```python
from build123d import *

# Parameters (mm, degrees)
F1_DEPTH = 44.45
F2_T     = -2.54
F4_DEPTH = 3.81
F5_R     = 4.205558
F6_DEPTH = 3.81


with BuildPart() as f1:
    # F0 (on Top) → F1 (new body)
    with BuildSketch(Plane.XY):
        with BuildLine():
            Line((40.64, 0), (0, 0))
            Line((0, 0), (0, -41.275))
            ThreePointArc((0, -41.275), (29.688681, -29.862048), (40.64, 0))
        make_face()
    extrude(amount=F1_DEPTH)

    # F2
    f2_openings = [f1.faces().sort_by_distance(p)[0] for p in [
        (0, -20.6375, 22.225),
        (20.32, 0, 22.225),
    ]]
    offset(amount=F2_T, openings=f2_openings)

    # F3 (on face) → F4 (join)
    with BuildSketch(Plane.XY.offset(44.45)):
        with BuildLine():
            ThreePointArc((0, -41.275), (29.688681, -29.862048), (40.64, 0))
            Line((40.64, 0), (31.781275, 0))
            Line((31.781275, 0), (22.916552, 0))
            Line((22.916552, 0), (0, 0))
            Line((0, 0), (0, -41.275))
        make_face()
        with BuildLine():
            Line((31.781275, 0), (40.64, 0))
            Line((40.64, 0), (40.64, 8.392821))
            ThreePointArc((40.64, 8.392821), (31.784439, 17.251546), (22.922552, 8.39915))
            Line((22.922552, 8.39915), (22.916552, 0))
            Line((22.916552, 0), (31.781275, 0))
        make_face()
        with BuildLine():
            ThreePointArc((35.966783, 8.392821), (34.740876, 5.43322), (31.781275, 4.207313))
            ThreePointArc((31.781275, 4.207313), (28.821674, 11.352422), (35.966783, 8.392821))
        make_face(mode=Mode.SUBTRACT)
    extrude(amount=F4_DEPTH)

    # F5 (on face) → F6 (join)
    with BuildSketch(Plane(origin=(0, 0, 0), x_dir=(1, 0, 0), z_dir=(0, 0, -1))):
        with BuildLine():
            Line((40.626373, -8.396372), (40.64, 0))
            Line((40.64, 0), (31.771399, 0))
            Line((31.771399, 0), (22.916414, 0))
            Line((22.916414, 0), (22.916414, -8.382))
            ThreePointArc((22.916414, -8.382), (31.764213, -17.236982), (40.626373, -8.396372))
        make_face()
        with Locations((31.771399, -8.382)):
            Circle(F5_R, mode=Mode.SUBTRACT)
        with BuildLine():
            Line((31.771399, 0), (40.64, 0))
            ThreePointArc((40.64, 0), (29.688681, 29.862048), (0, 41.275))
            Line((0, 41.275), (0, 0))
            Line((0, 0), (22.916414, 0))
            Line((22.916414, 0), (31.771399, 0))
        make_face()
    extrude(amount=F6_DEPTH)


solid = f1.part
```
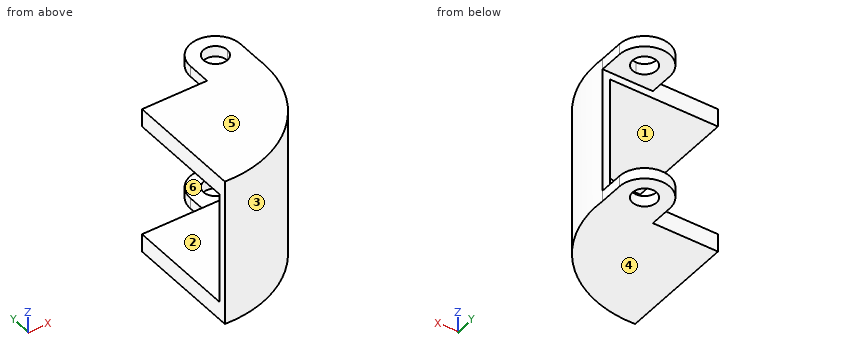
Can you work these out from the model? Positions are in its coordinate system, mm. Face numbers are marked on the shaded views. A direction names the side the tool comes from. Give positions to 0.01 mm unless a question says otherwise; leave off trailing zeros. Loops run counter-clockwise (first coordinate to the right, second up) from the corner with the lowest first, then second, coordinate; pieces in that order, holes last. Notation, with made-up numbers: M 11.25,5 L 46.25,5 A37 ccw 46.25,44 Z; hole C -5.5,81 d11. An arc over 180 degrees is marked long. Use one line per item in the form item = value. Start each with the question number.
(1) I want a section at B-B, the plane y = 5. Write out the boundary of the cut face in (x, z).
(2) I'm going to push flat-ended pins straight in: P1, Ø1.5, axis at x = 32.5, z = 25.5, coming from the +Y side; P2, Ø1.5, axis at x = 19, z = 38, coming from the -Y side; P3, Ø12, axis at y = -17, z = 28, coming from the +X side; P4, Ø5, axis at x = 34, y = 9, coming from the +Z side. Where does each tip first touch, or does it pass through?
(3) On a 3-axis mill with a long thin cutter (end or side, diameter ignored), from which of +Z, -Z, +X, -X, +Y, -Y can I reach the whole of each face in a straight line? I mean the marked faces 5 and 6. Say none if no direction works.
(4) I want a section at A-A, the plane x = 28.5. Write out the boundary of the cut face in (y, z).
(5) I want a section at C-C, the plane x = 13. Write out the boundary of the cut face in (y, z), and give its area (3 significant figures).
(6) Please list where these lines run through material, in increasing order: line 1 (Z direction, x = 2.5, y = -2.5); line 2 (Z direction, x = 23, y = 7); line 3 (Y direction, x = 28.5, z = 7.5).
(7) Thinking about a two-plate mould opening in Z: for the marked faces 1, 2, 3 and 4, which applies, released by +Z, released by -Z, zero draft, split by the parting line, or undercut?
(8) I want a section at D-D, the plane z = 1. Write out the boundary of the cut face in (x, y) (3 decimals), and give its area (3 significant figures).
Worked out:
q1.outline = M 22.92,-3.81 L 29.27,-3.81 L 29.27,0 L 22.92,0 Z; M 22.92,44.45 L 29.33,44.45 L 29.33,48.26 L 22.92,48.26 Z; M 34.23,44.45 L 40.64,44.45 L 40.64,48.26 L 34.23,48.26 Z; M 34.27,-3.81 L 40.63,-3.81 L 40.63,0 L 34.27,0 Z
q2.P1 = -21.08
q2.P2 = -37.87
q2.P3 = 39.88
q2.P4 = 48.26
q3.face_5 = +Z, +X, -X, +Y, -Y
q3.face_6 = +X, -X, +Y
q4.outline = M -31.02,-3.81 L 5.74,-3.81 L 5.74,0 L 0,0 L 0,2.54 L -27.43,2.54 L -27.43,41.91 L 0,41.91 L 0,44.45 L 5.79,44.45 L 5.79,48.26 L -31.02,48.26 Z; M 10.99,44.45 L 16.62,44.45 L 16.62,48.26 L 10.99,48.26 Z; M 11.02,-3.81 L 16.61,-3.81 L 16.61,0 L 11.02,0 Z
q5.outline = M -39.82,-3.81 L 0,-3.81 L 0,2.54 L -37.16,2.54 L -37.16,41.91 L 0,41.91 L 0,48.26 L -39.82,48.26 Z
q5.area = 610 mm²
q6.line_1 = -3.81 to 2.54, 41.91 to 48.26
q6.line_2 = -3.81 to 0, 44.45 to 48.26
q6.line_3 = -31.02 to -27.43
q7.face_1 = undercut
q7.face_2 = undercut
q7.face_3 = zero draft
q7.face_4 = released by -Z
q8.outline = M 0,-41.275 A38.473 ccw 40.64,0 L 0,0 Z
q8.area = 1,370 mm²
